from build123d import *
from build123d.topology import SkipClean

# Parameters (mm, degrees)
BOSS_EXTRUDE1_DEPTH = 76.2
SKETCH2_R           = 25.4
SKETCH2_R_2         = 4.0005
BOSS_EXTRUDE2_DEPTH = 101.6
SKETCH4_W           = 6.35
SKETCH4_H           = 19.05
SKETCH5_R           = 4.0005
CUT_EXTRUDE1_DEPTH  = 240.623120754
SKETCH7_R           = 10.9982
CUT_EXTRUDE2_DEPTH  = 239.462040028
CUT_EXTRUDE3_DEPTH  = 239.462040028


with BuildPart() as part:
    # Sketch1 → Boss-Extrude1 (new body)
    with BuildSketch(Plane.XY):
        Polygon((-203.2, 13.126834176), (-8.532442214, 13.126834176), (0, 0), (-203.2, 0), align=None)
        Polygon((119.24636491, 96.183058807), (-8.532442214, 13.126834176), (0, 0), (127.778807124, 83.056224631), align=None)
    extrude(amount=BOSS_EXTRUDE1_DEPTH)

    # Sketch2 → Boss-Extrude2 (add)
    with BuildSketch(Plane.XZ):
        with Locations(Location((-40.282442214, 38.1, 0), (0, 0, 270))):
            Circle(SKETCH2_R)
        with Locations((-40.282442214, 38.1)):
            Circle(SKETCH2_R_2, mode=Mode.SUBTRACT)
    extrude(amount=BOSS_EXTRUDE2_DEPTH)

    # Sketch4 → Cut-Revolve1 (revolve, cut)
    with BuildSketch(Plane.XY.offset(38.1), mode=Mode.PRIVATE) as cut_revolve1_sk:
        with Locations((-62.817567444, -32.3596)):
            Rectangle(SKETCH4_W, SKETCH4_H)
    revolve(cut_revolve1_sk.sketch.rotate(Axis((-40.282442214, -101.6, 38.1), (0, 1, 0)), 270), axis=Axis((-40.282442214, -101.6, 38.1), (0, 1, 0)), mode=Mode.SUBTRACT)

    # Sketch5 → Cut-Extrude1 (cut, through all)
    with SkipClean():  # the faces are left unmerged after this step: merging them gives an invalid solid
        with BuildSketch(Plane.XZ):
            with Locations(Location((-40.282442214, 38.1, 0), (0, 0, 90))):
                Circle(SKETCH5_R)
        extrude(amount=-CUT_EXTRUDE1_DEPTH, mode=Mode.SUBTRACT)

    # Sketch7 → Cut-Extrude2 (cut, through all)
    with SkipClean():  # the faces are left unmerged after this step: merging them gives an invalid solid
        with BuildSketch(Plane(origin=(-8.532442214, 13.126834176, 0), x_dir=(0.8384436163006369, 0.5449883505954145, 0), z_dir=(-0.5449883505954145, 0.838443616300637, 0))):
            with Locations(Location((61.0108, -38.1, 0), (0, 0, 180))):
                Circle(SKETCH7_R)
        extrude(amount=-CUT_EXTRUDE2_DEPTH, mode=Mode.SUBTRACT)

    # Sketch8 → Cut-Extrude3 (cut, through all)
    with SkipClean():  # the faces are left unmerged after this step: merging them gives an invalid solid
        with BuildSketch(Plane(origin=(-8.532442214, 13.126834176, 0), x_dir=(0.8384436163006369, 0.5449883505954145, 0), z_dir=(-0.5449883505954145, 0.838443616300637, 0))):
            with BuildLine():
                Line((76.2, 0), (152.4, 0))
                Line((152.4, 0), (152.4, -76.2))
                Line((152.4, -76.2), (76.2, -76.2))
                ThreePointArc((76.2, -76.2), (114.3, -38.1), (76.2, 0))
            make_face()
        extrude(amount=-CUT_EXTRUDE3_DEPTH, mode=Mode.SUBTRACT)


solid = part.part
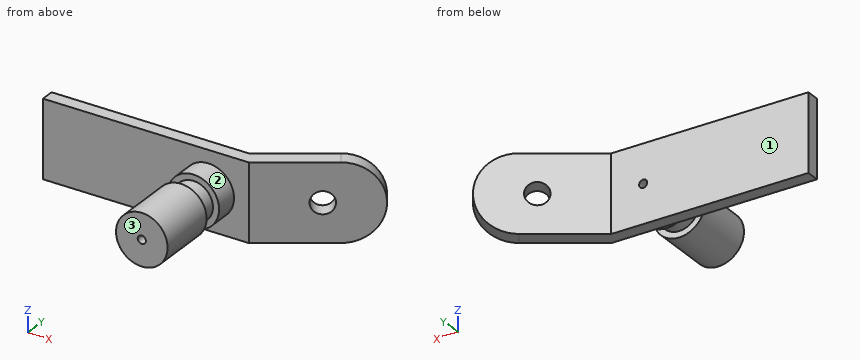
Input: part model. Units: mm. Frame: model coordinates. Face numbers are marked on the shaded views. A direction names the side the tool comes from. Round coordinates to 2 decimals unless told otherwise and drop trailing zeros. Order: outer loops, then holes, each group sorted by start corner. A loop starts at its lowest first (then second) coordinate and runs counter-clockwise, first axis right, second up. Notation, with made-up numbers: (62, 21) - (99, 21) arc R25 cw to (99, 47) - close; hole circle Ø2 at (10, 63.5). An arc over 180 degrees is marked (long way). Use a Markdown table: item, result.
1. Section C-C on z = 5. Return the cut outline in (x, y), then the cut area to 3 significant figures.
Evaluation:
| item | result |
|---|---|
| outline | (-203.2, 0) - (0, 0) - (79.71, 51.81) - (71.18, 64.94) - (-8.53, 13.13) - (-203.2, 13.13) - close |
| area | 4,100 mm^2 |
2. Section B-B on x = -73.5. Return the cut outline in (y, z), then the cut area to 3 significant figures.
Evaluation:
| item | result |
|---|---|
| outline | (0, 0) - (13.13, 0) - (13.13, 76.2) - (0, 76.2) - close |
| area | 1,000 mm^2 |
3. Section D-D on y = -27.5. Return the cut outline in (x, z), then the cut area to 3 significant figures.
Evaluation:
| item | result |
|---|---|
| outline | circle Ø38.72 at (-40.28, 38.1); hole circle Ø8 at (-40.28, 38.1) |
| area | 1,130 mm^2 |
4. First-contact query: pin 1 (2 mm diameter, centred on x = 23, z = 28, fed in from -Y); pin 2 (3 mm diameter, centred on y = 7.5, z = 24.5, fed in from +X); pin 3 (5 mm diameter, centred on y = 46, z = 52.5, fed in from -X); pin 4 (6.5 mm diameter, centred on x = -40.28, z = 38.1, fed in from -Y). Flat tips, straight axial feed; report the tip coordinate or a pass-through.
Evaluation:
| item | result |
|---|---|
| pin 1 | y = 14.3 |
| pin 2 | x = 13.85 |
| pin 3 | x = 38.2 |
| pin 4 | through |
5. Section A-A on z = 38.1. Return the cut outline in (x, y).
Evaluation:
| item | result |
|---|---|
| outline | (-203.2, 0) - (-65.68, 0) - (-65.68, -22.83) - (-59.64, -22.83) - (-59.64, -41.88) - (-65.68, -41.88) - (-65.68, -101.6) - (-44.28, -101.6) - (-44.28, 13.13) - (-203.2, 13.13) - close; (-36.28, -101.6) - (-14.88, -101.6) - (-14.88, -41.88) - (-20.92, -41.88) - (-20.92, -22.83) - (-14.88, -22.83) - (-14.88, 0) - (0, 0) - (41.93, 27.26) - (33.4, 40.38) - (-8.53, 13.13) - (-36.28, 13.13) - close; (51.84, 52.37) - (60.38, 39.24) - (95.83, 62.29) - (87.3, 75.42) - close |
6. Access query for the marked faces 1, 2 and 3. Directions: +Z, -Z, +X, -X, +Y, -Y. A direction counts if a zero-diameter tool reaches every point of the face in a straight line with its end or side. Return the directions, or none.
Evaluation:
| item | result |
|---|---|
| face 1 | +Z, -Z, -X, +Y |
| face 2 | -Y |
| face 3 | +Z, -Z, +X, -X, -Y |
7. Material intervals for probe 1 along X at (y, z) = (-59, 38.1); probe 2 along Y at (x, z) = (-42, 25.5); probe 3 along Y at (x, z) = (-94.5, 67), sorted ascending.
Evaluation:
| item | result |
|---|---|
| probe 1 | -65.68 to -44.28, -36.28 to -14.88 |
| probe 2 | -101.6 to 13.13 |
| probe 3 | 0 to 13.13 |
